```python
from build123d import *

# Parameters (mm, degrees)
F0_W     = 91
F0_H     = 12.5
F1_DEPTH = 42
F2_R     = 6


with BuildPart() as f1:
    # F0 (on Top) → F1 (new body)
    with BuildSketch(Plane.XY):
        Polygon((-26.282259, 45), (-26.282259, 0), (-17.682259, 0), (73.317741, 0), (80.717741, 0), (80.717741, 45), (27.717741, 45), (4.717741, 45), align=None)
        with Locations((27.817741, -6.25)):
            Rectangle(F0_W, F0_H)
        Polygon((11.217741, 73), (4.717741, 45), (27.717741, 45), (21.217741, 73), align=None)
    extrude(amount=F1_DEPTH)

    # F2
    f2_edges = [f1.edges().sort_by_distance(p)[0] for p in [
        (11.217741, 73, 21),
        (21.217741, 73, 21),
    ]]
    fillet(f2_edges, radius=F2_R)


solid = f1.part
```
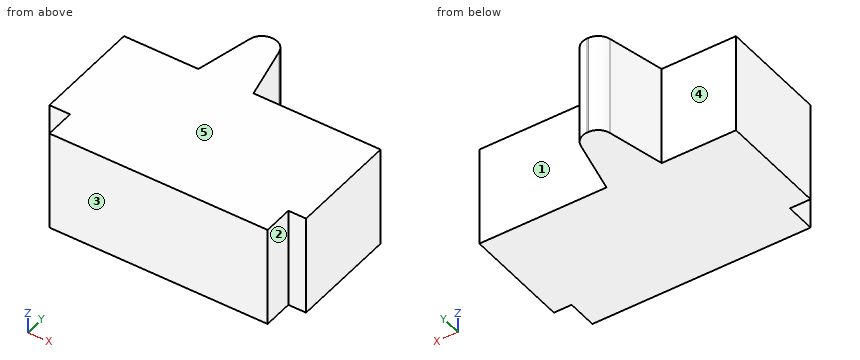
Verification items for the finished model (mm, model axes). Face numbers are marked on the shaded views. A direction names the side the tool comes from. Coordinates: 2 decimals unless noted, no trailing zeros. Order: outer loops, then holes, each group sorted by start corner. A loop starts at its lowest first (then second) coordinate and runs counter-clockwise, first axis right, second up. Notation, with made-up numbers: (67, -24.75) -> (76, -24.75) arc R10 cw to (76, -17.75) -> close; hole circle Ø7 at (62, 80). An arc over 180 degrees is marked (long way). Answer as CSV lines item,"result". Start each with the question number.
1) Gauge pin test, flat ends, axial feed: pin 1 Ø10 at (y, z) = (55.5, 25.5) entering from -X; pin 2 Ø10 at (y, z) = (-9.5, 27) entering from -X; pin 3 Ø6 at (x, y) = (30.5, 48.5) entering from +Z; pin 4 Ø7 at (x, z) = (-22.5, 26.5) entering from -Y. Record the tip position at first contact, or that the pin passes through.
2) Cross-section at A-A, the plane z = 38.5. Record the boundary of the cut face in (x, y).
3) Set-up check for the marked faces 1, 2, 3, 4 and 5: record each of +Z, -Z, +X, -X, +Y, -Y from which the full face is reachable in a straight line by a thin tool's end or side.
4) Material ranges on L1, parallel to Y at x = 64, z = 31.5; L2, parallel to Y at x = 73.5, z = 14.5; L3, parallel to X at y = -4, z = 20, recorded low to high. Write a range as [from, to].
5) Cross-section at C-C, the plane y = 57. Record the boundary of the cut face in (x, z).
6) Cross-section at B-B, the plane x = 47.5. Record the boundary of the cut face in (y, z), then the cut area to 4 significant figures.
Conclusion:
1,pin 1,"stops at x = 5.99"
1,pin 2,"stops at x = -17.68"
1,pin 3,"passes through"
1,pin 4,"stops at y = 0"
2,outline,"(-26.28, 0) -> (-17.68, 0) -> (-17.68, -12.5) -> (73.32, -12.5) -> (73.32, 0) -> (80.72, 0) -> (80.72, 45) -> (27.72, 45) -> (22.3, 68.36) arc R6 ccw to (16.45, 73) -> (15.98, 73) arc R6 ccw to (10.14, 68.36) -> (4.72, 45) -> (-26.28, 45) -> close"
3,face 1,"+Z, -Z, +X, +Y"
3,face 2,"+Z, -Z, +X, -Y"
3,face 3,"+Z, -Z, +X, -X, -Y"
3,face 4,"+Z, -Z, -X, +Y"
3,face 5,"+Z, +X, -X, +Y, -Y"
4,L1,"y = [-12.5, 45]"
4,L2,"y = [0, 45]"
4,L3,"x = [-17.68, 73.32]"
5,outline,"(7.5, 0) -> (24.93, 0) -> (24.93, 42) -> (7.5, 42) -> close"
6,outline,"(-12.5, 0) -> (45, 0) -> (45, 42) -> (-12.5, 42) -> close"
6,area,"2,415 mm²"
